Geometry: final body of the model. Coordinates: model frame, mm. A direction names the side the tool comes from. Give positions to 0.01 mm unless a question says otherwise; leave off trailing zeros. Order: outer loops, then holes, each group sorted by start corner. A loop starts at its lowest first (then second) coordinate and runs counter-clockwise, first axis right, second up. Notation, with made-up numbers: (26.5, -17.5) - (64.5, -17.5) arc R23 cw to (64.5, -9.5) - close; hole circle Ø11 at (-1.5, -11). An arc over 180 degrees is marked (long way). One line per item, written item: value.
```python
from build123d import *

# Parameters (mm, degrees)
SKETCH_W     = 23
SKETCH_H     = 9
PAD_DEPTH    = 30
SKETCH002_W  = 27
SKETCH002_H  = 12.5
PAD002_DEPTH = 2


with BuildPart() as display_hole_clone_body:
    # Sketch → Pad (new body)
    with BuildSketch(Plane.XY):
        with Locations((1.5, 0)):
            Rectangle(SKETCH_W, SKETCH_H)
    extrude(amount=PAD_DEPTH)


with BuildPart() as display_hole_clone_body_1:
    # Body placement: moved
    add(display_hole_clone_body.part.moved(Location((0, 0, -10))))


with BuildPart() as cut002:
    # Sketch002 → Pad002 (new body)
    with BuildSketch(Plane.XY):
        with Locations((1.5, 0)):
            Rectangle(SKETCH002_W, SKETCH002_H)
    extrude(amount=PAD002_DEPTH)

    # Cut002: cut display hole clone body
    add(display_hole_clone_body_1.part, mode=Mode.SUBTRACT)


solid = cut002.part
```
1) Material intervals for line 1 along X through (y, z) = (4, 0.75); line 2 along Y through (x, z) = (8.5, 1.5), sorted ascending.
Answers below:
line 1: -12 to -10, 13 to 15
line 2: -6.25 to -4.5, 4.5 to 6.25
2) Section C-C, the plane z = 0.9. Return loops of the section in (x, y).
Answers below:
outline: (-12, -6.25) - (15, -6.25) - (15, 6.25) - (-12, 6.25) - close; hole (-10, -4.5) - (13, -4.5) - (13, 4.5) - (-10, 4.5) - close
3) Section A-A, the plane y = 1.5. Return loops of the section in (x, z), then the cut area to 3 significant figures.
Answers below:
outline: (-12, 0) - (-10, 0) - (-10, 2) - (-12, 2) - close; (13, 0) - (15, 0) - (15, 2) - (13, 2) - close
area: 8.00 mm^2
4) Mould query, pull axis Y, two halves, no side actions, for faces 3 (the face through (1, 4.5, 1)), 4 (the face through (1, -6.25, 1)), 5 (the face through (-12, 0, 1)). Classes: released by +Y, released by -Y, zero draft, split by the parting line, or undercut.
Answers below:
face 3: undercut
face 4: released by -Y
face 5: zero draft
5) Section B-B, the plane x = -7.5. Return loops of the section in (y, z).
Answers below:
outline: (-6.25, 0) - (-4.5, 0) - (-4.5, 2) - (-6.25, 2) - close; (4.5, 0) - (6.25, 0) - (6.25, 2) - (4.5, 2) - close
6) Set-up query: faces 1 (the face through (1, 6.25, 1)), 2 (the face through (1, -4.5, 1)). Return all of +Z, -Z, +X, -X, +Y, -Y with unobstructed straight access to the full face (end or side cutting, diameter ignored); none if empty.
Answers below:
face 1: +Z, -Z, +X, -X, +Y
face 2: +Z, -Z
